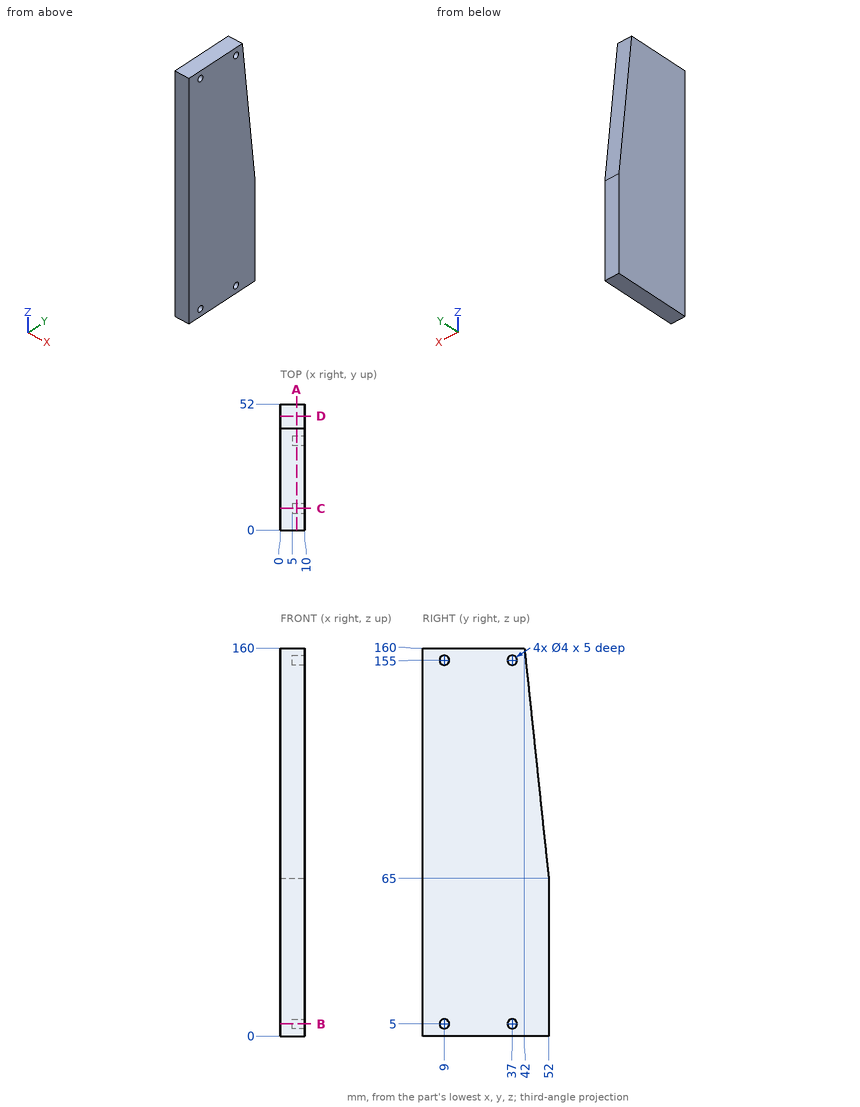
Here's the drawing with two shaded views (mm, measured from the low corner). I have some questions. Give positions to 0.01 mm unless a question says otherwise; leave off trailing zeros. Loops run counter-clockwise (first coordinate to the right, second up) from the corner with the lowest first, then second, coordinate; pieces in that order, holes last. Notation, with made-up numbers: M 82,51 L 132,51 A18 ccw 132,63 Z; hole C 18,26 d11. An arc over 180 degrees is marked long. Use one line per item in the form item = value. Start each with the question number.
(1) I want a section at D-D, the plane y = 47. Write out the boundary of the cut face in (x, z).
(2) I'm going to push flat-ended pins straight in: P1, Ø4.5, axis at y = 9, z = 156, coming from the +X side; P2, Ø1.2, axis at y = 36.5, z = 4, coming from the +X side. Where does each tip first touch, or does it pass through?
(3) Please list where these lines run through material, in increasing order: line 1 (Y direction, x = 8, z = 5); line 2 (Y direction, x = 6, z = 155); line 3 (Z direction, x = 5.25, y = 7.5).
(4) I want a section at B-B, the plane z = 5. Write out the boundary of the cut face in (x, y).
(5) I want a section at A-A, the plane x = 6.75. Write out the boundary of the cut face in (y, z), and give its area (3 significant figures).
(6) I want a section at C-C, the plane y = 9. Write out the boundary of the cut face in (x, z), and give its area (3 significant figures).
Worked out:
q1.outline = M 0,0 L 10,0 L 10,112.5 L 0,112.5 Z
q2.P1 = 10
q2.P2 = 5
q3.line_1 = 0 to 7, 11 to 35, 39 to 52
q3.line_2 = 0 to 7, 11 to 35, 39 to 42.53
q3.line_3 = 0 to 3.68, 6.32 to 153.68, 156.32 to 160
q4.outline = M 0,0 L 10,0 L 10,7 L 5,7 L 5,11 L 10,11 L 10,35 L 5,35 L 5,39 L 10,39 L 10,52 L 0,52 Z
q5.outline = M 0,0 L 52,0 L 52,65 L 42,160 L 0,160 Z; hole C 9,5 d4; hole C 9,155 d4; hole C 37,5 d4; hole C 37,155 d4
q5.area = 7,790 mm²
q6.outline = M 0,0 L 10,0 L 10,3 L 5,3 L 5,7 L 10,7 L 10,153 L 5,153 L 5,157 L 10,157 L 10,160 L 0,160 Z
q6.area = 1,560 mm²
